from build123d import *

# Parameters (mm, degrees)
EXTRUDE_1_DEPTH     = 2
SKETCH_2_R          = 1.6
CUT_EXTRUDE_1_DEPTH = 340.897900211
SKETCH_3_R          = 1.6
CUT_EXTRUDE_2_DEPTH = 340.897900211


with BuildPart() as part:
    # 草图1 → 凸台-拉伸1 (new body)
    with BuildSketch(Plane.XY):
        with BuildLine():
            Line((-58.97100696, 258.210702341), (211.02899304, 258.210702341))
            ThreePointArc((211.02899304, 258.210702341), (218.100060852, 255.281770153), (221.02899304, 248.210702341))
            Line((221.02899304, 248.210702341), (221.02899304, -141.789297659))
            ThreePointArc((221.02899304, -141.789297659), (218.100060852, -148.860365471), (211.02899304, -151.789297659))
            Line((211.02899304, -151.789297659), (-58.97100696, -151.789297659))
            ThreePointArc((-58.97100696, -151.789297659), (-66.042074772, -148.860365471), (-68.97100696, -141.789297659))
            Line((-68.97100696, -141.789297659), (-68.97100696, 248.210702341))
            ThreePointArc((-68.97100696, 248.210702341), (-66.042074772, 255.281770153), (-58.97100696, 258.210702341))
        make_face()
    extrude(amount=EXTRUDE_1_DEPTH)

    # 草图2 → 切除-拉伸1 (cut, through all)
    with BuildSketch(Plane.XY.offset(2)):
        with Locations((-64.97100696, 208.210702341)):
            Circle(SKETCH_2_R)
        with Locations((-64.97100696, 105.210702341)):
            Circle(SKETCH_2_R)
        with Locations((-64.97100696, 2.210702341)):
            Circle(SKETCH_2_R)
        with Locations((-64.97100696, -100.789297659)):
            Circle(SKETCH_2_R)
        with Locations((217.02899304, 208.210702341)):
            Circle(SKETCH_2_R)
        with Locations((217.02899304, 105.210702341)):
            Circle(SKETCH_2_R)
        with Locations((217.02899304, 2.210702341)):
            Circle(SKETCH_2_R)
        with Locations((217.02899304, -100.789297659)):
            Circle(SKETCH_2_R)
        with Locations((-50.97100696, 254.210702341)):
            Circle(SKETCH_2_R)
        with Locations((203.02899304, 254.210702341)):
            Circle(SKETCH_2_R)
        with Locations((-50.97100696, -147.789297659)):
            Circle(SKETCH_2_R)
        with Locations((76.02899304, -147.789297659)):
            Circle(SKETCH_2_R)
        with Locations((203.02899304, -147.789297659)):
            Circle(SKETCH_2_R)
    extrude(amount=-CUT_EXTRUDE_1_DEPTH, mode=Mode.SUBTRACT)

    # 草图3 → 切除-拉伸2 (cut, through all)
    with BuildSketch(Plane.XY.offset(2)):
        with Locations((33.02899304, 38.210702341)):
            Circle(SKETCH_3_R)
        with Locations((33.02899304, -49.789297659)):
            Circle(SKETCH_3_R)
        with Locations((-36.97100696, -49.789297659)):
            Circle(SKETCH_3_R)
        with Locations((-36.97100696, 38.210702341)):
            Circle(SKETCH_3_R)
        with BuildLine():
            Line((46.02899304, 56.210702341), (77.02899304, 56.210702341))
            ThreePointArc((77.02899304, 56.210702341), (81.978740508, 54.160449809), (84.02899304, 49.210702341))
            Line((84.02899304, 49.210702341), (84.02899304, 21.210702341))
            ThreePointArc((84.02899304, 21.210702341), (81.978740508, 16.260954873), (77.02899304, 14.210702341))
            Line((77.02899304, 14.210702341), (46.02899304, 14.210702341))
            ThreePointArc((46.02899304, 14.210702341), (41.079245572, 16.260954873), (39.02899304, 21.210702341))
            Line((39.02899304, 21.210702341), (39.02899304, 49.210702341))
            ThreePointArc((39.02899304, 49.210702341), (41.079245572, 54.160449809), (46.02899304, 56.210702341))
        make_face()
    extrude(amount=-CUT_EXTRUDE_2_DEPTH, mode=Mode.SUBTRACT)


solid = part.part
Verification items for the finished model (mm, model axes). Give positions to 0.01 mm unless a question says otherwise; leave off trailing zeros. Loops run counter-clockwise (first coordinate to the right, second up) from the corner with the lowest first, then second, coordinate; pieces in that order, holes last.
1) Thickness scan on line 1 along X through (y, z) = (35, 0.25); line 2 along Y through (x, z) = (75, 1.55); line 3 along Y through (x, z) = (43.5, 1.3). Record the ranges inside material, lowest first.
2) Sectioned sample at B-B, the plane z = 1.4. Count the separate pieces of the cut face and the enclosed holes in it, then the cut area to 3 significant figures.
3) Sectioned sample at A-A, the plane x = 53.5. Enter the section's corners in (y, z), then the cut area to 3 significant figures.
4) Depth check by flat-ended pin: pin 1 Ø4 at (x, y) = (127, 133.5) entering from -Z; pin 2 Ø3 at (x, y) = (217.03, 2.21) entering from +Z. Enter the tip coordinate at first touch or a pass-through.
Answers:
1. line 1: x = -68.97 to 39.03, 84.03 to 221.03
1. line 2: y = -151.79 to -149.01, -146.56 to 14.21, 56.21 to 258.21
1. line 3: y = -151.79 to 14.68, 55.74 to 258.21
2. separate pieces: 1
2. enclosed holes: 18
2. area: 117,000 mm2
3. outline: (-151.79, 0) - (14.21, 0) - (14.21, 2) - (-151.79, 2) - close; (56.21, 0) - (258.21, 0) - (258.21, 2) - (56.21, 2) - close
3. area: 736 mm2
4. pin 1: stops at z = 0
4. pin 2: passes through
